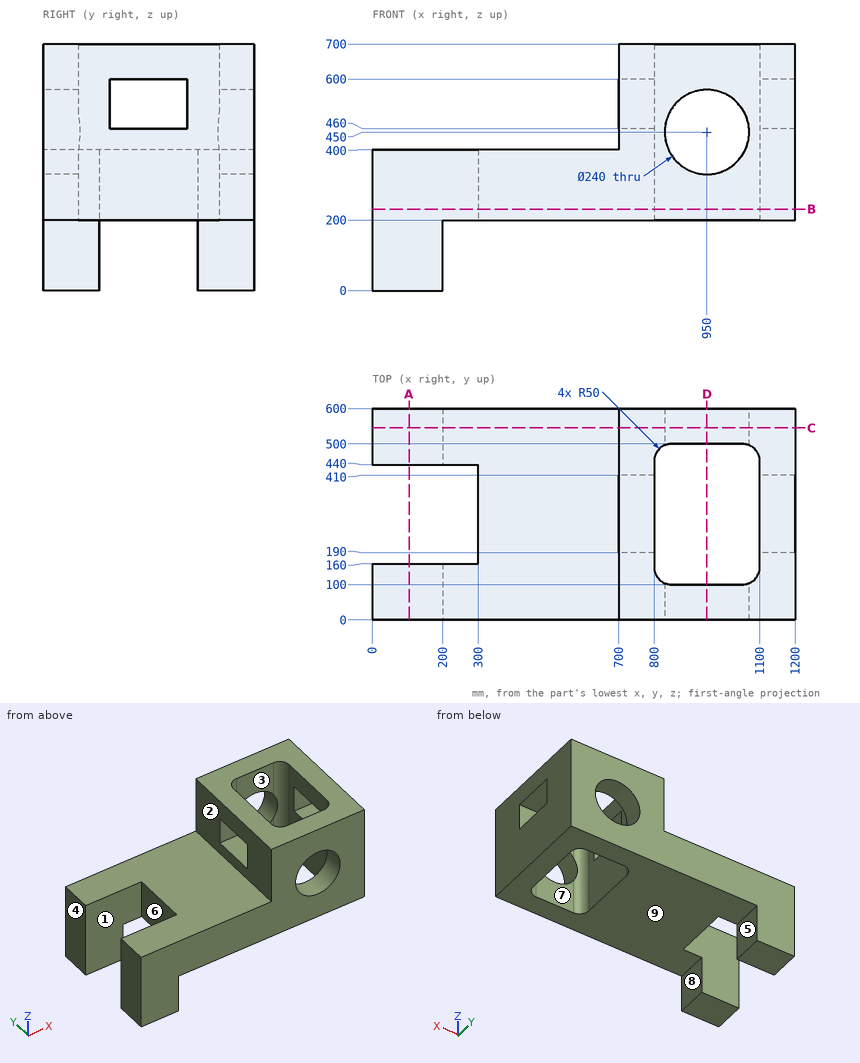
Could you check a few things on this drawing? It's one solid part, dimensions in mm from its lowest x, y, z. A direction names the side the tool comes from. Give positions to 0.01 mm unless a question says otherwise; leave off trailing zeros. Order: outer loops, then holes, each group sorted by start corner. A loop starts at its lowest first (then second) coordinate and runs counter-clockwise, first axis right, second up. Notation, with made-up numbers: (89.25, 51) - (148.25, 51) arc R16 ccw to (148.25, 82) - close; hole circle Ø3 at (0, 13.5). An arc over 180 degrees is marked (long way). Answer as a JSON object with one key per item and string values. Group by question number.
Item 1: If we section it at A-A on x = 104.5: Please give me the cut outline in (y, z).
Item 2: If we section it at D-D on x = 950: Please give me the cut outline in (y, z).
Item 3: Which directions (+Z, -Z, +X, -X, +Y, -Y) give clear straight access to the entire face, cutting with the end or side of a thin tool? Please do the marked faces 1, 2, 3, 4 and 5.
Item 4: Please list where these lines run through material, in increasing order: probe 1 along X at (y, z) = (557.5, 450); probe 2 along Z at (x, y) = (950, 34.5); probe 3 along X at (y, z) = (161.5, 418.5).
Item 5: If we section it at C-C on y = 545: Please give me the cut outline in (x, z).
Item 6: If we section it at B-B on z = 231.5: Please give me the cut outline in (x, y), and give its area (3 significant figures).
Item 7: For P1, Ø12, axis at x = 696.5, y = 212, coming from the -Z side; P2, Ø1, axis at y = 344, z = 296.5, coming from the -X side; P3, Ø4, axis at y = 412.5, z = 609.5, coming from the -X side, each with a flat end and sliding along its axis, tell me the tip position at first contact or that it passes through.
Item 8: If we mould it in two halves opening along X, with no side actions, what happens to the marked faces 6, 7, 8 and 9? For each: pulls with the +X half, pulls with the -X half, needs draft (parallel to the pull), parting line crosses it, or undercut.
Result set:
{
 "1": {"outline": "(0, 0) - (160, 0) - (160, 400) - (0, 400) - close; (440, 0) - (600, 0) - (600, 400) - (440, 400) - close"},
 "2": {"outline": "(0, 200) - (100, 200) - (100, 330) - (0, 330) - close; (0, 570) - (100, 570) - (100, 700) - (0, 700) - close; (500, 200) - (600, 200) - (600, 330) - (500, 330) - close; (500, 570) - (600, 570) - (600, 700) - (500, 700) - close"},
 "3": {"face 1": "+Z, -Z, -X", "face 2": "+Z, -X, +Y, -Y", "face 3": "+Z, -Z", "face 4": "+Z, -Z, -X, +Y, -Y", "face 5": "-Z, +X, +Y, -Y"},
 "4": {"probe 1": "700 to 830, 1070 to 1200", "probe 2": "200 to 330, 570 to 700", "probe 3": "700 to 800, 1100 to 1200"},
 "5": {"outline": "(0, 0) - (200, 0) - (200, 200) - (1200, 200) - (1200, 700) - (700, 700) - (700, 400) - (0, 400) - close; hole circle Ø240 at (950, 450)"},
 "6": {"outline": "(0, 0) - (1200, 0) - (1200, 600) - (0, 600) - (0, 440) - (300, 440) - (300, 160) - (0, 160) - close; hole (800, 150) arc R50 ccw to (850, 100) - (1050, 100) arc R50 ccw to (1100, 150) - (1100, 450) arc R50 ccw to (1050, 500) - (850, 500) arc R50 ccw to (800, 450) - close", "area": "518,000 mm²"},
 "7": {"P1": "z = 200", "P2": "x = 300", "P3": "x = 700"},
 "8": {"face 6": "pulls with the -X half", "face 7": "undercut", "face 8": "pulls with the +X half", "face 9": "needs draft"}
}
